Verification items for this drawing (mm, ordinates from the low corner). A direction names the side the tool comes from. Give positions to 0.01 mm unless a question says otherwise; leave off trailing zeros. Order: outer loops, then holes, each group sorted by start corner. A loop starts at its lowest first (then second) coordinate and runs counter-clockwise, first axis right, second up.
(1) Sectioned sample at D-D on x = 1.5. Record the cut outline in (y, z).
(2) Sectioned sample at B-B on x = 4. Record the cut outline in (y, z).
(3) Gauge pin test, flat end, axial feed: pin 1 (0.6 mm diameter, centred on x = 4, z = 1.5, fed in from -Y). Record the tip position at first contact, or that the pin passes through.
(4) Scan lines: L1, parallel to X at y = 3, z = 1.3; L2, parallel to Y at x = 2.75, z = 2.9 (1 decimal); L3, parallel to X at y = 19.5, z = 2.5. Record each from-to range of solid material in increasing order.
(5) Sectioned sample at C-C on z = 1. Record the cut outline in (x, y).
(6) Mould release check, pull along Y, two halves, no side actions. Record for the marked faces 4, 5, 6 and 7: pulls with the +Y half, pulls with the -Y half, needs draft (parallel to the pull), parting line crosses it, or undercut.
(7) Access from +Z, -Z, +X, -X, +Y, -Y to the whole of each face (thin tool, end or side, straight path). Record for the marked faces 1, 2 and 3.
(8) Sectioned sample at A-A on y = 2.25. Record the cut outline in (x, z).
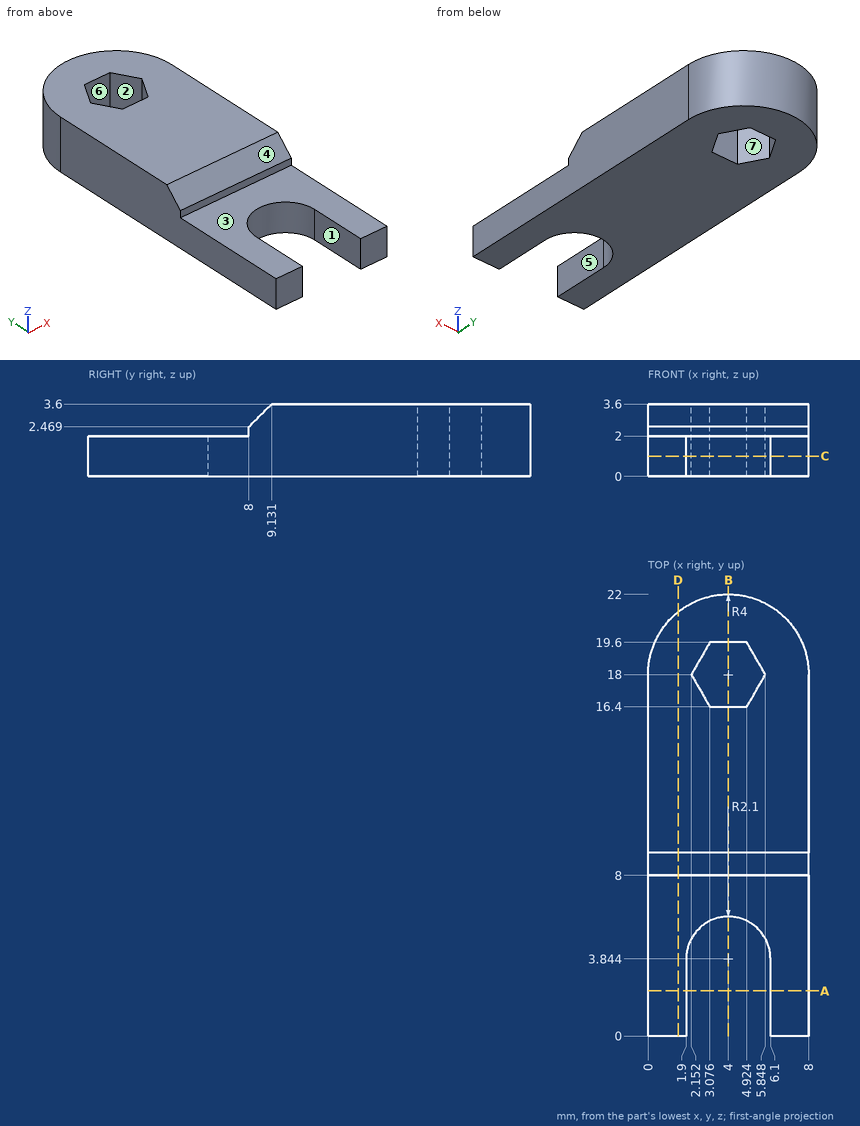
Ans:
1. outline: (0, 0) - (21.12, 0) - (21.12, 3.6) - (9.13, 3.6) - (8, 2.47) - (8, 2) - (0, 2) - close
2. outline: (5.94, 0) - (16.4, 0) - (16.4, 3.6) - (9.13, 3.6) - (8, 2.47) - (8, 2) - (5.94, 2) - close; (19.6, 0) - (22, 0) - (22, 3.6) - (19.6, 3.6) - close
3. pin 1: stops at y = 5.92
4. L1: x = 0 to 1.9, 6.1 to 8
4. L2: y = 8.4 to 17, 19 to 21.8
4. L3: x = 0.29 to 3.02, 4.98 to 7.71
5. outline: (0, 0) - (1.9, 0) - (1.9, 3.84) arc R2.1 cw to (6.1, 3.84) - (6.1, 0) - (8, 0) - (8, 18) arc R4 ccw to (0, 18) - close; hole (2.15, 18) - (3.08, 16.4) - (4.92, 16.4) - (5.85, 18) - (4.92, 19.6) - (3.08, 19.6) - close
6. face 4: pulls with the -Y half
6. face 5: needs draft
6. face 6: undercut
6. face 7: undercut
7. face 1: +Z, -Z, -Y
7. face 2: +Z, -Z
7. face 3: +Z, +X, -X, -Y
8. outline: (0, 0) - (1.9, 0) - (1.9, 2) - (0, 2) - close; (6.1, 0) - (8, 0) - (8, 2) - (6.1, 2) - close
